Input: part model. Units: mm. Frame: model coordinates. A direction names the side the tool comes from. Coordinates: 2 decimals unless noted, no trailing zeros. Loops run counter-clockwise (first coordinate to the right, second up) from the corner with the lowest first, then second, coordinate; pieces in that order, holes last. Notation, with made-up numbers: (67, 74.5) - (103, 74.5) arc R20 ccw to (103, 90.5) - close; hole circle Ø4 at (19.5, 4.5). An arc over 180 degrees is marked (long way). Use one line per item in the form item = value.
Autodesk Inventor part; units mm, degrees
ref_plane "YZ Plane" through (0, 0, 0) normal (1, 0, 0) x (0, 1, 0)
ref_plane "XZ Plane" through (0, 0, 0) normal (0, 1, 0) x (-1, 0, 0)
ref_plane "XY Plane" through (0, 0, 0) normal (0, 0, 1) x (1, 0, 0)
sketch "Sketch1" plane through (0, 0, 0) normal (0, 0, 1) x (1, 0, 0)
  line L0 (0, 0) -> (12, 0)
  line L1 (12, 0) -> (12, 4)
  line L2 (12, 4) -> (8.15, 4)
  line L3 (8.15, 4) -> (7.15, 3.84)
  line L4 (7.15, 3.84) -> (6.2, 3.84)
  line L5 (5.9, 4.52) -> (4.65, 4.52)
  line L6 (4.65, 4.52) -> (1.27, 7.9)
  line L7 (1.27, 7.9) -> (0, 7.9)
  line L8 (0, 7.9) -> (0, 0)
  line L9 (5.9, 4.52) -> (5.9, 4.14)
  arc A0 (5.9, 4.14) -> (6.2, 3.84) centre (6.2, 4.14) ccw
  dimension "d17" = 12
  dimension "d18" = 1.27
  dimension "d19" = 4.65
  dimension "d20" = 1.25
  dimension "d21" = 15.8
  dimension "d22" = 8
  dimension "d23" = 7.68
  dimension "d25" = 45
  dimension "d26" = 1
  dimension "d28" = 0.3
  dimension "d29" = 3.85
  dimension "d30" = 0.3
  dimension "d52" = 3.5
revolve "Revolution1" add sketch "Sketch1" angle 360 about axis through (0, 0, 0) along (1, 0, 0)
thread "Thread1"
sketch "Sketch2" plane through (0, 0, 0) normal (-1, 0, 0) x (0, 0, 1)
  circle A0 centre (0, 0) radius 3.975 construction
  circle A1 centre (0, 0) radius 2.7825 construction
  line L0 (0, 0) -> (2.4097, 1.3913)
  line L1 (0, 0) -> (2.7825, 0) construction
  line L2 (0, 0) -> (2.4097, -1.3912)
  line L3 (0, 0) -> (2.7825, 0) construction
  line L4 (2.4097, 1.3913) -> (3.975, 0)
  line L5 (3.975, 0) -> (2.4097, -1.3912)
  dimension "d34" = 7.95
  dimension "d35" = 5.565
  dimension "d39" = 30
  dimension "d40" = 330
extrude "Extrusion1" cut sketch "Sketch2" against normal blind 2.54
pattern_circular "Circular Pattern1" count 6 over 360 about axis through (-10, 0, 0) along (1, 0, 0) of "Extrusion1"
fillet "Fillet1" radius 0.8 12 edges at (1.27, 1.3913, 2.4097) (1.27, 0, 3.975) (1.27, -1.3912, 2.4097) (1.27, -2.7825, 0) (1.27, -3.4425, 1.9875) (1.27, -3.4425, -1.9875) (1.27, -1.3912, -2.4097) (1.27, 0, -3.975) (1.27, 1.3912, -2.4097) (1.27, 3.4425, -1.9875) (1.27, 2.7825, 0) (1.27, 3.4425, 1.9875)
equation "\"d17\" = l_"
equation "\"d18\" = 0.5 * t"
equation "\"d19\" = k"
equation "\"d20\" = shldr"
equation "\"d21\" = dk"
equation "\"d22\" = d"
equation "\"d23\" = ds_"
equation "\"d25\" = 0.5 * headAngle"
equation "\"d26\" = x"
equation "\"d28\" = r"
equation "\"d29\" = b"
equation "\"d32\" = b"
equation "\"d34\" = A_"
equation "\"d35\" = 0.7 * A_"
equation "\"d43\" = t"
equation "\"d48\" = v"
equation "\"A_\" = 7.95"
equation "\"t\" = 2.54"
equation "\"v\" = 0.1 * d"
equation "\"dk\" = 15.8"
equation "\"k\" = 4.65"
equation "\"l_\" = 12"
equation "\"shldr\" = 1.25"
equation "\"d\" = 8"
equation "\"p\" = 0.8"
equation "\"x\" = 1"
equation "\"ds_\" = 0.96 * d"
equation "\"headAngle\" = 90deg"
equation "\"c_\" = 0.35 * v"
equation "\"r\" = 0.3"
properties part number "Vite a testa svasata piana incassata esalobulare ISO 14581 - M8x12-4.8" material "Acciaio"
Q1. Set-up query: faces 1 (the cylindrical face through (6.668, 3.663, -1.153)), 2 (the cylindrical face through (5.266, -0.98, 4.413)), 3 (the cylindrical face through (1.29, 3.09, -1.79)). Return all of +Z, -Z, +X, -X, +Y, -Y with unobstructed straight access to the full face (end or side cutting, diameter ignored); none if empty.
Check values:
face_1 = none
face_2 = +X
face_3 = -X
Q2. Pull-direction query (Z, two-part tool) for faces 4 (the flat face through (0, 3, 0)), 5 (the cylindrical face through (1.29, -3.09, 1.79)), 6 (the conical face through (4.439, -4.727, -0.208)); classes: pulls with the +Z half, pulls with the -Z half, needs draft (parallel to the pull), parting line crosses it, or undercut.
Check values:
face_4 = needs draft
face_5 = undercut
face_6 = parting line crosses it
Q3. Cut plane B-B, the plane z = 0. Return loops of the section in (x, y).
Check values:
outline = (0, -7.9) - (1.27, -7.9) - (4.65, -4.52) - (5.9, -4.52) - (5.9, -4.14) arc R0.3 cw to (6.2, -3.84) - (7.15, -3.84) - (8.15, -4) - (12, -4) - (12, 4) - (8.15, 4) - (7.15, 3.84) - (6.2, 3.84) arc R0.3 cw to (5.9, 4.14) - (5.9, 4.52) - (4.65, 4.52) - (1.27, 7.9) - (0, 7.9) - (0, 2.83) - (2.54, 2.83) - (2.54, -2.83) - (0, -2.83) - close
Q4. Cut plane D-D, the plane x = 9.5. Return loops of the section in (y, z), then the cut area to 3 significant figures.
Check values:
outline = circle Ø8 at (0, 0)
area = 50.3 mm²
Q5. First-contact query: P1, Ø6, axis at x = 5.5, y = -4.5, coming from the +Z side; P2, Ø2, axis at y = 3, z = 4.5, coming from the -X side; P3, Ø5, axis at x = 8.5, y = -3, coming from the +Z side; P4, Ø1.5, axis at y = -4.5, z = 4.5, coming from the +X side. Flat tips, straight axial feed; report the tip coordinate or a pass-through.
Check values:
P1 = 5.51
P2 = 0
P3 = 3.97
P4 = 3.56
Q6. Cut plane C-C, the plane x = 4.25. Return loops of the section in (y, z), then the cut area to 3 significant figures.
Check values:
outline = circle Ø9.84 at (0, 0)
area = 76.0 mm²
Q7. Ray query, line 1 along Y through (x, z) = (1.5, 3.25); line 2 along Z through (x, y) = (2, -0.75); line 3 along X through (y, z) = (-2.25, -4.5). Return the intervals inside material, ascending. Write a range as [from, to].
Check values:
line_1 = [-6.95, -0.64], [0.64, 6.95]
line_2 = [-7.13, -3.13], [3.13, 7.13]
line_3 = [0, 4.14]
Q8. Cut plane A-A, the plane y = 0. Return loops of the section in (x, z), then the cut area to 3 significant figures.
Check values:
outline = (0, -7.9) - (1.27, -7.9) - (4.65, -4.52) - (5.9, -4.52) - (5.9, -4.14) arc R0.3 cw to (6.2, -3.84) - (7.15, -3.84) - (8.15, -4) - (12, -4) - (12, 4) - (8.15, 4) - (7.15, 3.84) - (6.2, 3.84) arc R0.3 cw to (5.9, 4.14) - (5.9, 4.52) - (4.65, 4.52) - (1.27, 7.9) - (0, 7.9) - (0, 3.57) - (2.54, 3.57) - (2.54, -3.57) - (0, -3.57) - close
area = 103 mm²
